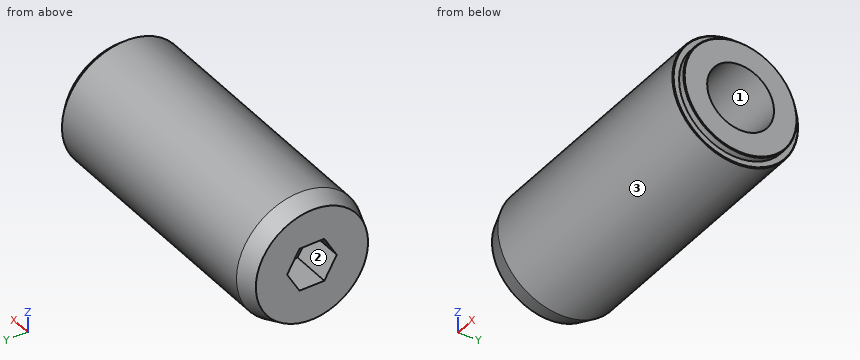
from build123d import *

# Parameters (mm, degrees)
CORTAR_EXTRUIR1_DEPTH      = 5
CHAFL_N1_SIZE              = 0.1
TALADRO_ROSCADO_M101_D     = 8.5
TALADRO_ROSCADO_M101_DEPTH = 25
TALADRO_ROSCADO_M101_TIP   = 2.553657631


with BuildPart() as part:
    # Sketch1 → Revolve1 (revolve)
    with BuildSketch(Plane.XY, mode=Mode.PRIVATE) as revolve1_sk:
        Polygon((-3, 7.99722512), (-35.734329665, 7.99722512), (-38.096725725, 7.137383273), (-38.096725725, -0.00277488), (-2.096725725, -0.00277488), (-2.096725725, 7.2074675), (-3, 7.2074675), align=None)
    revolve(revolve1_sk.sketch.rotate(Axis((-38.096725725, -0.00277488, 0), (1, 0, 0)), 180), axis=Axis((-38.096725725, -0.00277488, 0), (1, 0, 0)))

    # Croquis3 → Cortar-Extruir1 (cut)
    with BuildSketch(Plane.ZY.offset(38.096725725)):
        Polygon((0, -3.156760752), (2.733835005, -1.578380376), (2.733835005, 1.578380376), (0, 3.156760752), (-2.733835005, 1.578380376), (-2.733835005, -1.578380376), align=None)
    extrude(amount=-CORTAR_EXTRUIR1_DEPTH, mode=Mode.SUBTRACT)

    # Chaflán1
    chafl_n1_edges = [part.edges().sort_by_distance(p)[0] for p in [
        (-2.096725725, 7.2074675, 0),
        (-3, 7.99722512, 0),
    ]]
    chamfer(chafl_n1_edges, length=CHAFL_N1_SIZE)

    # Taladro roscado M101
    with Locations(Plane(origin=(-2.096725725, 0, 0), x_dir=(0, 0, -1), z_dir=(1, 0, 0))):
        with Locations((0, 0)):
            Hole(TALADRO_ROSCADO_M101_D / 2, depth=TALADRO_ROSCADO_M101_DEPTH)
            with Locations((0, 0, -(TALADRO_ROSCADO_M101_DEPTH + TALADRO_ROSCADO_M101_TIP / 2))):  # 118° drill point
                Cone(0, TALADRO_ROSCADO_M101_D / 2, TALADRO_ROSCADO_M101_TIP, mode=Mode.SUBTRACT)


solid = part.part
Design review of the part built by this model. Coordinates are the model's own, in mm. Face numbers are marked on the shaded views. A direction names the side the tool comes from. Coordinates: 2 decimals unless noted, no trailing zeros. Order: outer loops, then holes, each group sorted by start corner. A loop starts at its lowest first (then second) coordinate and runs counter-clockwise, first axis right, second up. Notation, with made-up numbers: M -8,-14.5 L -1,-14.5 A9 cw -1,1.5 Z; hole C -29.75,-17.5 d7. An arc over 180 degrees is marked long. Use a Markdown table: item, result.
(1) For the marked faces 1, 2 and 3, list the 3-axis set-ups (+Z, -Z, +X, -X, +Y, -Y) from which the entire face can be reached by the end or side of a thin tool; tool diameter is ignored.
Worked answers:
| item | result |
|---|---|
| face 1 | +X |
| face 2 | -X |
| face 3 | +X, -X |
(2) Add section B-B (x = -29). Give the boundary of the cut face in (y, z), then the cut area to 3 significant figures.
Worked answers:
| item | result |
|---|---|
| outline | C 0,0 d16; hole C 0,0 d2.16 |
| area | 197 mm2 |
(3) Add section A-A (x = -11.5). Give the boundary of the cut face in (y, z), then the cut area to 3 significant figures.
Worked answers:
| item | result |
|---|---|
| outline | C 0,0 d16; hole C 0,0 d8.5 |
| area | 144 mm2 |
(4) For P1, Ø4, axis at x = -12, y = -4, coming from the -Z side; P2, Ø4, axis at x = -20.5, y = 4.5, coming from the +Z side; P3, Ø4, axis at x = -15.5, z = -5, coming from the -Y side, all flat-tipped, find the tip position at first contact; note any pin that passes through.
Worked answers:
| item | result |
|---|---|
| P1 | stops at z = -7.75 |
| P2 | stops at z = 7.6 |
| P3 | stops at y = -7.42 |
(5) Wall thickness on probe 1 along Z at (x, y) = (-17.75, 0); probe 2 along Y at (x, z) = (-10.5, 3.5); probe 3 along Z at (x, y) = (-32.5, 3.75): over which ranges is each line inside the solid? List them lowest first.
Worked answers:
| item | result |
|---|---|
| probe 1 | z = -8 to -4.25, 4.25 to 8 |
| probe 2 | y = -7.2 to -2.41, 2.41 to 7.19 |
| probe 3 | z = -7.07 to 7.07 |
